from build123d import *

# Parameters (mm, degrees)
SKETCH_1_R      = 5
SKETCH_1_R_2    = 1.7
EXTRUDE_1_DEPTH = 2.2


with BuildPart() as part:
    # 草图1 → 凸台-拉伸1 (new body)
    with BuildSketch(Plane(origin=(0, 0, 0), x_dir=(1, 0, 0), z_dir=(0, 1, 0))):
        with BuildLine():
            Line((14.611038219, -6.7), (49.690443214, -6.7))
            Line((49.690443214, -6.7), (59.14213471, -6.376451123))
            ThreePointArc((59.14213471, -6.376451123), (62.116009682, 1.036036266), (57.195522798, 7.327118086))
            add(Edge.make_bspline(
                [(50.347107534, 9.880159683), (52.761361064, 9.443859829), (55.044166152, 8.592845964), (57.195522798, 7.327118086)],
                knots=[0.288436631, 0.288436631, 0.288436631, 0.288436631, 1, 1, 1, 1], degree=3))
            add(Edge.make_bspline(
                [(41.984360593, 6.514151987), (43.667045792, 8.848960271), (46.317081673, 10.55679372), (49.303704664, 10.196073302), (50.347107534, 9.880159683)],
                knots=[0.090085046, 0.090085046, 0.090085046, 0.090085046, 0.520368733, 0.736118782, 0.736118782, 0.736118782, 0.736118782], degree=3))
            add(Edge.make_bspline(
                [(18.29395406, 7.037125327), (29.823970963, -0.449921726), (41.984360593, 6.514151987)],
                knots=[0, 0, 0, 1, 1, 1], degree=2))
            add(Edge.make_bspline(
                [(6.555128163, 14.676604942), (13.508953417, 12.492816522), (18.29395406, 7.037125327)],
                knots=[0, 0, 0, 1, 1, 1], degree=2))
            ThreePointArc((6.555128163, 14.676604942), (2.774471684, 15.832711225), (-1.174023286, 16.031035749))
            add(Edge.make_bspline(
                [(-4.132506817, 15.533667476), (-4.311159294, 25.643963381), (-1.174023286, 16.031035749)],
                knots=[0, 0, 0, 1, 1, 1], degree=2))
            add(Edge.make_bspline(
                [(-6.029547406, 14.900234761), (-4.764310754, 14.268430824), (-4.132506817, 15.533667476)],
                knots=[0, 0, 0, 1, 1, 1], degree=2))
            add(Edge.make_bspline(
                [(-8.69333509, 13.520294481), (-11.961242179, 23.089556901), (-6.029547406, 14.900234761)],
                knots=[0, 0, 0, 1, 1, 1], degree=2))
            add(Edge.make_bspline(
                [(-10.305043141, 12.336065974), (-8.907074862, 12.122326202), (-8.69333509, 13.520294481)],
                knots=[0, 0, 0, 1, 1, 1], degree=2))
            add(Edge.make_bspline(
                [(-12.417884822, 10.206300721), (-18.460681491, 18.31398895), (-10.305043141, 12.336065974)],
                knots=[0, 0, 0, 1, 1, 1], degree=2))
            add(Edge.make_bspline(
                [(-13.589217783, 8.585196439), (-12.192999161, 8.810082099), (-12.417884822, 10.206300721)],
                knots=[0, 0, 0, 1, 1, 1], degree=2))
            add(Edge.make_bspline(
                [(-15.07242577, 5.585196439), (-23.295073991, 11.517146599), (-13.589217783, 8.585196439)],
                knots=[0, 0, 0, 1, 1, 1], degree=2))
            add(Edge.make_bspline(
                [(-15.669039675, 3.585196439), (-14.412461062, 4.29933734), (-15.07242577, 5.585196439)],
                knots=[0, 0, 0, 1, 1, 1], degree=2))
            add(Edge.make_bspline(
                [(-16.063311706, 0.585196439), (-25.780917218, 3.388231532), (-15.669039675, 3.585196439)],
                knots=[0, 0, 0, 1, 1, 1], degree=2))
            add(Edge.make_bspline(
                [(-16.011582331, -1.414803561), (-15.037875075, -0.394118455), (-16.063311706, 0.585196439)],
                knots=[0, 0, 0, 1, 1, 1], degree=2))
            add(Edge.make_bspline(
                [(-15.455806267, -4.414803561), (-25.566384923, -4.736394924), (-16.011582331, -1.414803561)],
                knots=[0, 0, 0, 1, 1, 1], degree=2))
            add(Edge.make_bspline(
                [(-14.787919584, -6.299989859), (-14.179269776, -5.023453369), (-15.455806267, -4.414803561)],
                knots=[0, 0, 0, 1, 1, 1], degree=2))
            add(Edge.make_bspline(
                [(-13.318124412, -9), (-22.835991784, -12.431149783), (-14.787919584, -6.299989859)],
                knots=[0, 0, 0, 1, 1, 1], degree=2))
            ThreePointArc((-13.318124412, -9), (1.319244681, -16.019738803), (14.611038219, -6.7))
        make_face()
        with Locations(Location((0, 0, 0), (0, 0, 270))):
            Circle(SKETCH_1_R, mode=Mode.SUBTRACT)
        with Locations(Location((0, 8.4, 0), (0, 0, 270))):
            Circle(SKETCH_1_R_2, mode=Mode.SUBTRACT)
        with Locations(Location((8.4, 0, 0), (0, 0, 270))):
            Circle(SKETCH_1_R_2, mode=Mode.SUBTRACT)
        with Locations(Location((-8.4, 0, 0), (0, 0, 270))):
            Circle(SKETCH_1_R_2, mode=Mode.SUBTRACT)
        with Locations(Location((0, -8.4, 0), (0, 0, 270))):
            Circle(SKETCH_1_R_2, mode=Mode.SUBTRACT)
    extrude(amount=EXTRUDE_1_DEPTH)


solid = part.part
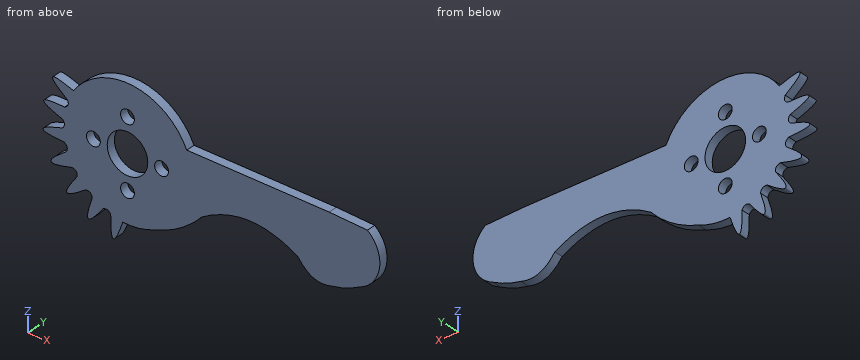
Check sheet for the modelled part. Datum: model origin and axes. Units: mm. Coordinates: 2 decimals unless noted, no trailing zeros. Write item = value, one per line. Start each with the question number.
1. Material ranges on line 1 (X direction, y = 1.55, z = 0); line 2 (X direction, y = 0.9, z = -8.4); line 3 (Z direction, x = 0.5, y = 2), recorded low to high.
2. Section check A-A on y = 1.45. Give the number of separate pieces and of enclosed holes in the cut face, then the cut area to 3 significant figures.
3. Depth check by flat-ended pin: P1, Ø1.5, axis at x = 52.5, z = -8.5, coming from the -Y side; P2, Ø2.5, axis at x = 0, z = 8.4, coming from the +Y side; P3, Ø1.1, axis at x = 36.5, y = 1.5, coming from the +Z side. Enter the tip coordinate at first touch or a pass-through.
Responses:
q1.line_1 = -15.63 to -10.1, -6.7 to -5, 5 to 6.7, 10.1 to 62.2
q1.line_2 = -18.44 to -1.7, 1.7 to 17.01, 43.63 to 55.12
q1.line_3 = -16.07 to -10.02, -6.78 to -4.97, 4.97 to 6.78, 10.02 to 16.07
q2.separate_pieces = 1
q2.enclosed_holes = 5
q2.area = 1,370 mm2
q3.P1 = 0
q3.P2 = through
q3.P3 = 6.7
